Here's how the part is built. I have some questions about the finished solid (model axes, mm). Coordinates: 2 decimals unless noted, no trailing zeros. Loops run counter-clockwise (first coordinate to the right, second up) from the corner with the lowest first, then second, coordinate; pieces in that order, holes last. Notation, with made-up numbers: (64, 10) -> (98, 10) arc R16 ccw to (98, 38) -> close; hole circle Ø3 at (45.5, 61). An arc over 180 degrees is marked (long way). Answer as a JSON object with one key per item and string values. Group by question number.
1) I want a section at A-A (x = -17). Write out the boundary of the cut face in (y, z).
2) I want a section at C-C (y = 10.59). Write out the boundary of the cut face in (x, z).
3) I want a section at B-B (z = 0.7). Write out the boundary of the cut face in (x, y), then the cut area to 3 significant figures.
4) I want a section at D-D (x = 2.5). Write out the boundary of the cut face in (y, z).
5) I need wall thicknesses on probe 1 along Y at (x, z) = (-36.77, 0.5); probe 2 along X at (y, z) = (8.5, 0.9); probe 3 along X at (y, z) = (9.25, 0.8). Which ranges of each line are inside material? Lowest first, please. Write a range as [from, to].
```python
from build123d import *

# Parameters (mm, degrees)
F0_R     = 1.5875
F1_DEPTH = 1
F2_R     = 1.625
F2_R_2   = 2
F2_R_3   = 6
F2_W     = 14
F2_H     = 14
F2_W_2   = 23.3
F2_H_2   = 14.8
F2_W_3   = 13
F2_H_3   = 9.9
F3_DEPTH = 1.001
F7_DEPTH = 1.001


with BuildPart() as f1:
    # F0 (on Top) → F1 (new body)
    with BuildSketch(Plane.XY):
        with BuildLine():
            Line((-53.6, -21.2), (53.6, -21.2))
            ThreePointArc((53.6, -21.2), (55.014214, -20.614214), (55.6, -19.2))
            Line((55.6, -19.2), (55.6, -10.9))
            ThreePointArc((55.6, -10.9), (55.746447, -10.546447), (56.1, -10.4))
            Line((56.1, -10.4), (61.2, -10.4))
            ThreePointArc((61.2, -10.4), (64.278275, -9.506617), (66.4, -7.104078))
            Line((66.4, -7.104078), (66.4, -2.195922))
            ThreePointArc((66.4, -2.195922), (64.278275, 0.206617), (61.2, 1.1))
            Line((61.2, 1.1), (56.1, 1.1))
            ThreePointArc((56.1, 1.1), (55.746447, 1.246447), (55.6, 1.6))
            Line((55.6, 1.6), (55.6, 9.9))
            ThreePointArc((55.6, 9.9), (55.014214, 11.314214), (53.6, 11.9))
            Line((53.6, 11.9), (28.895582, 11.9))
            ThreePointArc((28.895582, 11.9), (25.215973, 12.358319), (21.761222, 13.70527))
            Line((21.761222, 13.70527), (11.238778, 19.39473))
            ThreePointArc((11.238778, 19.39473), (7.784027, 20.741681), (4.104418, 21.2))
            Line((4.104418, 21.2), (-50.6, 21.2))
            ThreePointArc((-50.6, 21.2), (-54.135534, 19.735534), (-55.6, 16.2))
            Line((-55.6, 16.2), (-55.6, -19.2))
            ThreePointArc((-55.6, -19.2), (-55.014214, -20.614214), (-53.6, -21.2))
        make_face()
        with Locations((-52.1, -17.7)):
            Circle(F0_R, mode=Mode.SUBTRACT)
        with Locations((61.2, -4.65)):
            Circle(F0_R, mode=Mode.SUBTRACT)
        with Locations((-52.1, 17.7)):
            Circle(F0_R, mode=Mode.SUBTRACT)
    extrude(amount=F1_DEPTH)

    # F2 (on face) → F3 (cut, through all)
    with BuildSketch(Plane.XY.offset(1)):
        with Locations((-47.02, 13.84)):
            Circle(F2_R)
        with Locations((-47.02, -15.16)):
            Circle(F2_R)
        with Locations((-40.02, -12.66)):
            Circle(F2_R_2)
        with Locations((-32.72, -12.66)):
            Circle(F2_R_2)
        with Locations((-36.77, 10.59)):
            Circle(F2_R_3)
        with Locations((3.03, 10.59)):
            Circle(F2_R_3)
        with Locations((-11.22, 10.54)):
            Rectangle(F2_W, F2_H)
        with Locations((-18.02, -10.86)):
            Rectangle(F2_W_2, F2_H_2)
        with Locations((-2.32, -12.66)):
            Circle(F2_R_2)
        with Locations((4.98, -12.66)):
            Circle(F2_R_2)
        with Locations((11.98, -15.16)):
            Circle(F2_R)
        with Locations((11.98, 13.84)):
            Circle(F2_R)
        with BuildLine():
            Line((37.656189, -4.65), (48.356189, -4.65))
            ThreePointArc((48.356189, -4.65), (43.006189, 0.7), (37.656189, -4.65))
        make_face()
        with Locations((25.482554, -9.6)):
            Rectangle(F2_W_3, F2_H_3)
        with Locations((25.482554, 0.3)):
            Rectangle(F2_W_3, F2_H_3)
        with BuildLine():
            ThreePointArc((37.656189, -4.65), (43.006189, -10), (48.356189, -4.65))
            Line((48.356189, -4.65), (37.656189, -4.65))
        make_face()
    extrude(amount=-F3_DEPTH, mode=Mode.SUBTRACT)

    # F6 (on face) → F7 (intersect, through all)
    with BuildSketch(Plane.XY.offset(1)):
        with BuildLine():
            Line((3.03, 20.09), (-36.77, 20.09))
            ThreePointArc((-36.77, 20.09), (-41.528618, 18.81226), (-45.007177, 15.322749))
            ThreePointArc((-45.007177, 15.322749), (-44.636923, 13.08439), (-46.229309, 11.468332))
            ThreePointArc((-46.229309, 11.468332), (-43.791188, 4.190553), (-36.77, 1.09))
            Line((-36.77, 1.09), (3.03, 1.09))
            ThreePointArc((3.03, 1.09), (10.025937, 4.162958), (12.495933, 11.393817))
            ThreePointArc((12.495933, 11.393817), (9.630133, 12.986696), (10.806132, 16.047268))
            ThreePointArc((10.806132, 16.047268), (7.41212, 19.01894), (3.03, 20.09))
        make_face()
    extrude(amount=-F7_DEPTH, mode=Mode.INTERSECT)


solid = f1.part
```
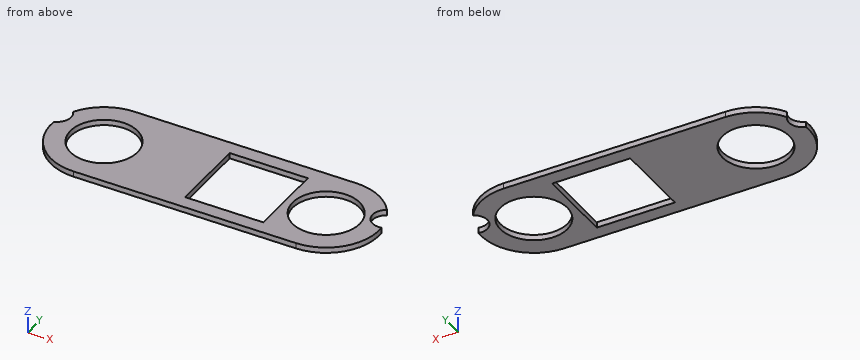
Determined:
{
 "1": {"outline": "(1.09, 0) -> (3.54, 0) -> (3.54, 1) -> (1.09, 1) -> close; (17.54, 0) -> (20.09, 0) -> (20.09, 1) -> (17.54, 1) -> close"},
 "2": {"outline": "(-46.27, 0) -> (-42.77, 0) -> (-42.77, 1) -> (-46.27, 1) -> close; (-30.77, 0) -> (-18.22, 0) -> (-18.22, 1) -> (-30.77, 1) -> close; (-4.22, 0) -> (-2.97, 0) -> (-2.97, 1) -> (-4.22, 1) -> close; (9.03, 0) -> (12.53, 0) -> (12.53, 1) -> (9.03, 1) -> close"},
 "3": {"outline": "(-46.23, 11.47) arc R9.5 ccw to (-36.77, 1.09) -> (3.03, 1.09) arc R9.5 ccw to (12.5, 11.39) arc R2.5 cw to (10.81, 16.05) arc R9.5 ccw to (3.03, 20.09) -> (-36.77, 20.09) arc R9.5 ccw to (-45.01, 15.32) arc R2.5 cw to start; hole circle Ø12 at (-36.77, 10.59); hole (-18.22, 3.54) -> (-4.22, 3.54) -> (-4.22, 17.54) -> (-18.22, 17.54) -> close; hole circle Ø12 at (3.03, 10.59)", "area": "605 mm^2"},
 "4": {"outline": "(1.09, 0) -> (4.61, 0) -> (4.61, 1) -> (1.09, 1) -> close; (16.57, 0) -> (20.09, 0) -> (20.09, 1) -> (16.57, 1) -> close"},
 "5": {"probe 1": "[1.09, 4.59], [16.59, 20.09]", "probe 2": "[-46.04, -42.39], [-31.15, -18.22], [-4.22, -2.59], [8.65, 12.3]", "probe 3": "[-46.18, -42.62], [-30.92, -18.22], [-4.22, -2.82], [8.88, 12.44]"}
}
